```python
from build123d import *

# Parameters (mm, degrees)
F0_W      = 5.3952559829
F0_H      = 21.7885393649
F0_W_2    = 6.4328089356
F0_H_2    = 60.9454013749
F1_DEPTH  = 12.5
F2_R      = 3
F2_R_2    = 3.25
F2_R_3    = 3.5
F2_R_4    = 4
F2_R_5    = 4.5
F2_R_6    = 5
F2_R_7    = 5.5
F3_DEPTH  = 65.591439771
F4_W      = 25
F4_H      = 62.590439771
F5_DEPTH  = 146.2136954069
F6_DEPTH  = 25
F7_W      = 3
F7_H      = 15
F7_W_2    = 50
F7_H_2    = 1.2136954069
F8_DEPTH  = 3
F9_R      = 4
F9_R_2    = 3.75
F9_R_3    = 3.5
F9_R_4    = 3.25
F9_R_5    = 3
F9_R_6    = 2.75
F9_R_7    = 2.5
F9_R_8    = 2.25
F10_DEPTH = 3


with BuildPart() as f1:
    # F0 (on Right) → F1 (new body, symmetric)
    with BuildSketch(Plane.YZ):
        with Locations((-29.570158571, 3.008893691)):
            Rectangle(F0_W, F0_H)
        Polygon((113.9459088445, 18.5482017696), (-32.2677865624, 18.5482017696), (-32.2677865624, 13.9031633735), (-26.8725305796, 13.9031633735), (107.5130999088, 13.9031633735), (113.9459088445, 13.9031633735), align=None)
        with Locations((110.7295043766, -16.569537314)):
            Rectangle(F0_W_2, F0_H_2)
    extrude(amount=F1_DEPTH, both=True)

    # F2 (on face) → F3 (cut, through all)
    with BuildSketch(Plane.XY.offset(18.5482017696)):
        with Locations((0, -28.0540911555)):
            Circle(F2_R)
        with Locations((0, -20.0540911555)):
            Circle(F2_R)
        with Locations((0, -12.0540911555)):
            Circle(F2_R_2)
        with Locations((0, -4.0540911555)):
            Circle(F2_R_2)
        with Locations((0, 3.9459088445)):
            Circle(F2_R_3)
        with Locations((0, 12.9459088445)):
            Circle(F2_R_3)
        with Locations((0, 21.9459088445)):
            Circle(F2_R_4)
        with Locations((0, 31.9459088445)):
            Circle(F2_R_4)
        with Locations((0, 41.9459088445)):
            Circle(F2_R_5)
        with Locations((0, 52.9459088445)):
            Circle(F2_R_5)
        with Locations((0, 64.9459088445)):
            Circle(F2_R_6)
        with Locations((0, 76.9459088445)):
            Circle(F2_R_6)
        with Locations((0, 89.9459088445)):
            Circle(F2_R_7)
        with Locations((0, 103.9459088445)):
            Circle(F2_R_7)
    extrude(amount=-F3_DEPTH, mode=Mode.SUBTRACT)

    # F4 (on face) → F5 (cut, through all)
    with BuildSketch(Plane(origin=(0, 113.9459088445, 0), x_dir=(-1, 0, 0), z_dir=(0, 1, 0))):
        with Locations((0, -15.7470181159)):
            Rectangle(F4_W, F4_H)
    extrude(amount=-F5_DEPTH, mode=Mode.SUBTRACT)

    # F6 (add): a face of the model
    f6_faces = [f1.faces().sort_by_distance(p)[0] for p in [
        (-12.5, 40.839061141, 17.0482017696),
    ]]
    extrude(f6_faces, amount=F6_DEPTH)

    # F7 (on face) → F8 (cut, through all)
    with BuildSketch(Plane.XY.offset(18.5482017696)):
        with Locations((-36, -9.7677865624)):
            Rectangle(F7_W, F7_H)
        with Locations((-36, 15.2322134376)):
            Rectangle(F7_W, F7_H)
        with Locations((-36, 40.2322134376)):
            Rectangle(F7_W, F7_H)
        with Locations((-36, 65.2322134376)):
            Rectangle(F7_W, F7_H)
        with Locations((-36, 90.2322134376)):
            Rectangle(F7_W, F7_H)
        with Locations((-12.5, 113.339061141)):
            Rectangle(F7_W_2, F7_H_2)
    extrude(amount=-F8_DEPTH, mode=Mode.SUBTRACT)

    # F9 (on face) → F10 (cut, through all)
    with BuildSketch(Plane.XY.offset(18.5482017696)):
        with Locations((-22.5, 102.7322134376)):
            Circle(F9_R)
        with Locations((-22.5, 92.2322134376)):
            Circle(F9_R)
        with Locations((-22.5, 82.2322134376)):
            Circle(F9_R_2)
        with Locations((-22.5, 72.2322134376)):
            Circle(F9_R_2)
        with Locations((-22.5, 62.2322134376)):
            Circle(F9_R_3)
        with Locations((-22.5, 52.2322134376)):
            Circle(F9_R_3)
        with Locations((-22.5, 43.2322134376)):
            Circle(F9_R_4)
        with Locations((-22.5, 34.2322134376)):
            Circle(F9_R_4)
        with Locations((-22.5, 26.2322134376)):
            Circle(F9_R_5)
        with Locations((-22.5, 18.2322134376)):
            Circle(F9_R_5)
        with Locations((-22.5, 10.2322134376)):
            Circle(F9_R_6)
        with Locations((-22.5, 2.2322134376)):
            Circle(F9_R_6)
        with Locations((-22.5, -4.7677865624)):
            Circle(F9_R_7)
        with Locations((-22.5, -11.7677865624)):
            Circle(F9_R_7)
        with Locations((-22.5, -17.7677865624)):
            Circle(F9_R_8)
        with Locations((-22.5, -23.7677865624)):
            Circle(F9_R_8)
    extrude(amount=-F10_DEPTH, mode=Mode.SUBTRACT)


solid = f1.part
```
The model under review builds one solid part; all positions refer to its coordinate system, in mm. A direction names the side the tool comes from. Round coordinates to 2 decimals unless told otherwise and drop trailing zeros.
Item 1: For pin 1 (0.9 mm diameter, centred on y = 16.5, z = 17.5, fed in from -X), flat-tipped, find the tip position at first contact; note if it passes through.
Working result:
pin 1: stops at x = -34.5
Item 2: To check wall thickness, follow probe 1 along X at (y, z) = (4, 18.2); probe 2 along X at (y, z) = (10.5, 18.4). State the ranges of each line that lie inside material, in increasing order.
Working result:
probe 1: x = -37.5 to -24.61, -20.39 to -3.5, 3.5 to 12.5
probe 2: x = -34.5 to -25.24, -19.76 to -2.5, 2.5 to 12.5
Item 3: Machinability: for faces 4 (the cylindrical face through (-24.881, 24.407, 17.069)), 5 (the flat face through (-36, 47.732, 17)), which of the approach directions +Z, -Z, +X, -X, +Y, -Y give a long, thin tool a straight path to every point of the face, cutting with its end or side? Answer none if there is none.
Working result:
face 4: +Z, -Z
face 5: +Z, -Z, -X
Item 4: Add section A-A, the plane x = -22.5. Count the separate pieces of the cut face and the enclosed holes in it, and give its area (3 significant figures).
Working result:
separate pieces: 17
enclosed holes: 0
area: 135 mm2
Item 5: Draft analysis for pull direction Y (two halves, no side actions). For faces 1 (the flat face through (-13, 112.732, 17)), 2 (the flat face through (12.5, 39, 17)), 3 (the flat face through (-34.5, -10, 17)), state which applies: released by +Y, released by -Y, zero draft, split by the parting line, or undercut.
Working result:
face 1: released by +Y
face 2: zero draft
face 3: undercut
